Can you work these out from the model? Positions are in its coordinate system, mm. A direction names the side the tool comes from. Round coordinates to 2 decimals unless told otherwise and drop trailing zeros. Loops run counter-clockwise (first coordinate to the right, second up) from the corner with the lowest first, then second, coordinate; pieces in that order, holes last.
```python
from build123d import *

# Parameters (mm, degrees)
F0_W     = 27.686
F0_H     = 27.686
F1_DEPTH = 647.7
F2_W     = 22.86
F2_H     = 22.86
F3_DEPTH = 635
F5_DEPTH = 56.134
F6_W     = 8.5673183203
F6_H     = 89.4483327866
F7_DEPTH = 68.326


with BuildPart() as f1:
    # F0 (on Top) → F1 (new body)
    with BuildSketch(Plane.XY):
        Rectangle(F0_W, F0_H)
    extrude(amount=F1_DEPTH)

    # F2 (on face) → F3 (cut)
    with BuildSketch(Plane.XY.offset(647.7)):
        Rectangle(F2_W, F2_H)
    extrude(amount=-F3_DEPTH, mode=Mode.SUBTRACT)

    # F4 (on face) → F5 (cut)
    with BuildSketch(Plane.YZ.offset(13.843)):
        with BuildLine():
            ThreePointArc((0, 628.65), (-4.4901280605, 630.5098719395), (-6.35, 635))
            Line((-6.35, 635), (-6.35, 323.85))
            Line((-6.35, 323.85), (0, 323.85))
            Line((0, 323.85), (0, 628.65))
        make_face()
        with BuildLine():
            Line((0, 628.65), (0, 635))
            Line((0, 635), (-6.35, 635))
            ThreePointArc((-6.35, 635), (-4.4901280605, 630.5098719395), (0, 628.65))
        make_face()
        with BuildLine():
            Line((0, 635), (0, 641.35))
            ThreePointArc((0, 641.35), (-4.4901280605, 639.4901280605), (-6.35, 635))
            Line((-6.35, 635), (0, 635))
        make_face()
        with BuildLine():
            ThreePointArc((6.35, 635), (4.4901280605, 639.4901280605), (0, 641.35))
            Line((0, 641.35), (0, 635))
            Line((0, 635), (6.35, 635))
        make_face()
        with BuildLine():
            Line((6.35, 635), (0, 635))
            Line((0, 635), (0, 628.65))
            ThreePointArc((0, 628.65), (4.4901280605, 630.5098719395), (6.35, 635))
        make_face()
        with BuildLine():
            Line((6.35, 323.85), (6.35, 635))
            ThreePointArc((6.35, 635), (4.4901280605, 630.5098719395), (0, 628.65))
            Line((0, 628.65), (0, 323.85))
            Line((0, 323.85), (6.35, 323.85))
        make_face()
        with BuildLine():
            Line((0, 323.85), (-6.35, 323.85))
            Line((-6.35, 323.85), (-6.35, 19.05))
            ThreePointArc((-6.35, 19.05), (-4.4901280605, 23.5401280605), (0, 25.4))
            Line((0, 25.4), (0, 323.85))
        make_face()
        with BuildLine():
            Line((6.35, 19.05), (6.35, 323.85))
            Line((6.35, 323.85), (0, 323.85))
            Line((0, 323.85), (0, 25.4))
            ThreePointArc((0, 25.4), (4.4901280605, 23.5401280605), (6.35, 19.05))
        make_face()
        with BuildLine():
            ThreePointArc((0, 12.7), (4.4901280605, 14.5598719395), (6.35, 19.05))
            Line((6.35, 19.05), (0, 19.05))
            Line((0, 19.05), (0, 12.7))
        make_face()
        with BuildLine():
            Line((0, 19.05), (-6.35, 19.05))
            ThreePointArc((-6.35, 19.05), (-4.4901280605, 14.5598719395), (0, 12.7))
            Line((0, 12.7), (0, 19.05))
        make_face()
        with BuildLine():
            ThreePointArc((0, 25.4), (-4.4901280605, 23.5401280605), (-6.35, 19.05))
            Line((-6.35, 19.05), (0, 19.05))
            Line((0, 19.05), (0, 25.4))
        make_face()
        with BuildLine():
            Line((0, 19.05), (6.35, 19.05))
            ThreePointArc((6.35, 19.05), (4.4901280605, 23.5401280605), (0, 25.4))
            Line((0, 25.4), (0, 19.05))
        make_face()
    extrude(amount=-F5_DEPTH, mode=Mode.SUBTRACT)

    # F6 (on face) → F7 (cut)
    with BuildSketch(Plane.XZ.offset(13.843)):
        with Locations((0, 534.5633029938)):
            Rectangle(F6_W, F6_H)
    extrude(amount=-F7_DEPTH, mode=Mode.SUBTRACT)


solid = f1.part
```
(1) We'd pull the mould along Y, two halves only. Please class faces 3 (the flat face through (0, 13.843, 319)), 4 (the flat face through (0, 0, 0)), 5 (the flat face through (-11.43, -8, 335)): released by +Y, released by -Y, zero draft, split by the parting line, or undercut.
(2) Suppose I cut it at A-A (z = 523). Write out the boundary of the cut face in (x, y).
(3) Suppose I cut it at B-B (z = 106). Write out the boundary of the cut face in (x, y), then the cut area to 3 significant figures.
(4) Which directions (+Z, -Z, +X, -X, +Y, -Y) give clear straight access to the entire face, cutting with the end or side of a thin tool? Please do faces 1 (the flat face through (0, -11.43, 335)), 2 (the flat face through (13.843, -9, 319)).
(5) If I drill on line 1 (X direction, y = -11, z = 88); line 2 (Z direction, x = 12.5, y = 1.25), over which ranges is the centre line in solid material (lowest first)?
(6) For pin 1 (2 mm diameter, centred on x = -9, y = 6, fed in from +Z), with a flat end and sliding along its axis, tell me the tip position at first contact or that it passes through.
Check result:
1. face 3: released by +Y
1. face 4: zero draft
1. face 5: undercut
2. outline: (-13.84, -13.84) - (-4.28, -13.84) - (-4.28, -11.43) - (-11.43, -11.43) - (-11.43, -6.35) - (-13.84, -6.35) - close; (-13.84, 6.35) - (-11.43, 6.35) - (-11.43, 11.43) - (-4.28, 11.43) - (-4.28, 13.84) - (-13.84, 13.84) - close; (4.28, -13.84) - (13.84, -13.84) - (13.84, -6.35) - (11.43, -6.35) - (11.43, -11.43) - (4.28, -11.43) - close; (4.28, 11.43) - (11.43, 11.43) - (11.43, 6.35) - (13.84, 6.35) - (13.84, 13.84) - (4.28, 13.84) - close
3. outline: (-13.84, -13.84) - (13.84, -13.84) - (13.84, -6.35) - (11.43, -6.35) - (11.43, -11.43) - (-11.43, -11.43) - (-11.43, -6.35) - (-13.84, -6.35) - close; (-13.84, 6.35) - (-11.43, 6.35) - (-11.43, 11.43) - (11.43, 11.43) - (11.43, 6.35) - (13.84, 6.35) - (13.84, 13.84) - (-13.84, 13.84) - close
3. area: 183 mm2
4. face 1: +Z
4. face 2: +Z, -Z, +X, +Y, -Y
5. line 1: x = -13.84 to -11.43, 11.43 to 13.84
5. line 2: z = 0 to 12.82, 641.23 to 647.7
6. pin 1: stops at z = 12.7
